The figure shows three views and two pictorial views of one solid part (mm, origin at its lowest corner). Answer the questions. Round coordinates to 2 decimals unless told otherwise and drop trailing zeros. Write each loop counter-clockwise with the first axis right and the second up, starting at its lowest first coordinate (ties: lowest second). Pieces come first, ordered by that corner, then holes. Notation, with made-up numbers: M 29,24.5 L 68,24.5 A26 cw 68,42.5 Z; hole C 17.5,41.25 d8. An arc over 180 degrees is marked long. Answer in a Markdown table with one row per item.
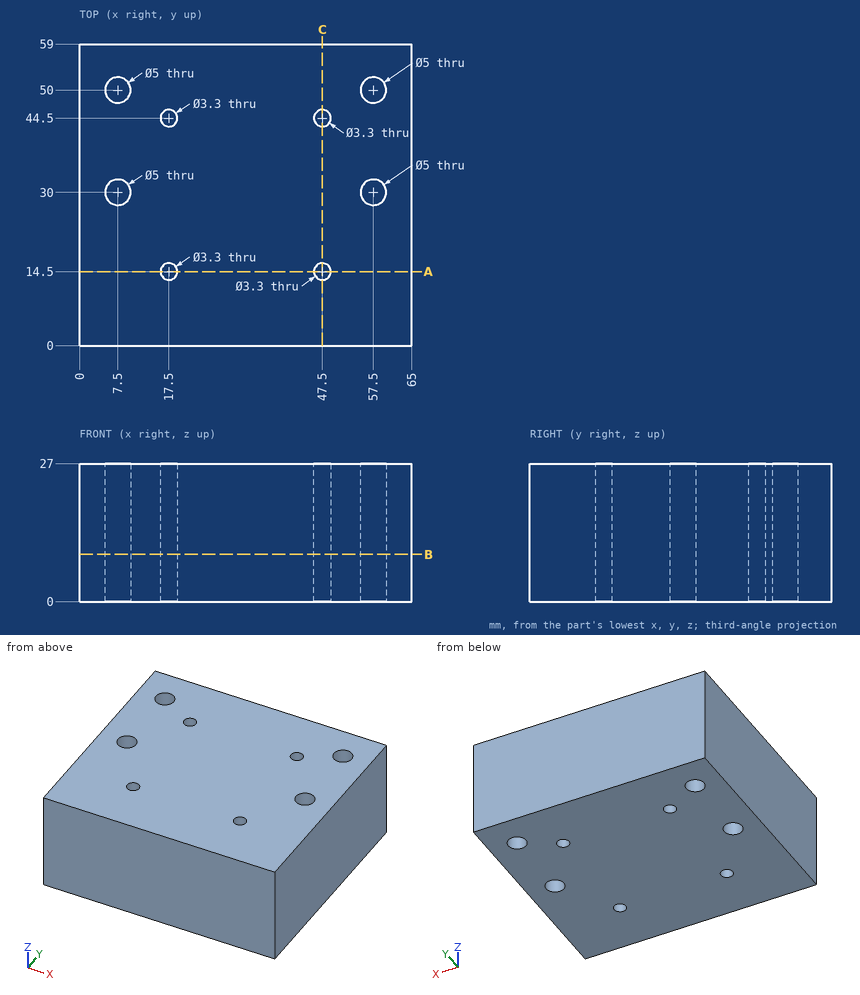
1. Consider line 1 along Y through (x, z) = (47.5, 9.75); line 2 along Y through (x, z) = (7.5, 13); line 3 along X through (y, z) = (48, 23.25). Determine where each line is inside the solid, lowest interval first. Write a range as from..to.
Calculated:
| item | result |
|---|---|
| line 1 | y = 0..12.85, 16.15..42.85, 46.15..59 |
| line 2 | y = 0..27.5, 32.5..47.5, 52.5..59 |
| line 3 | x = 0..6, 9..56, 59..65 |
2. The part is cut by section B-B (z = 9.25). Count the separate pieces of the cut face and the enclosed holes in it, plus the area to 3 significant figures.
Calculated:
| item | result |
|---|---|
| separate pieces | 1 |
| enclosed holes | 8 |
| area | 3,720 mm² |
3. Given pin 1 (4 mm diameter, centred on x = 7.5, y = 50, fed in from -Z), flat-ended and moving along its own axis, determine where the tip first touches the part or whether it passes through.
Calculated:
| item | result |
|---|---|
| pin 1 | passes through |
4. The part is cut by section A-A (y = 14.5). Determine the outline of the cut face in (x, z), plus the area to 3 significant figures.
Calculated:
| item | result |
|---|---|
| outline | M 0,0 L 15.85,0 L 15.85,27 L 0,27 Z; M 19.15,0 L 45.85,0 L 45.85,27 L 19.15,27 Z; M 49.15,0 L 65,0 L 65,27 L 49.15,27 Z |
| area | 1,580 mm² |
5. The part is cut by section C-C (x = 47.5). Determine the outline of the cut face in (y, z).
Calculated:
| item | result |
|---|---|
| outline | M 0,0 L 12.85,0 L 12.85,27 L 0,27 Z; M 16.15,0 L 42.85,0 L 42.85,27 L 16.15,27 Z; M 46.15,0 L 59,0 L 59,27 L 46.15,27 Z |
